Here's the drawing with two shaded views (mm, measured from the low corner). I have some questions. Coordinates: 2 decimals unless noted, no trailing zeros. Loops run counter-clockwise (first coordinate to the right, second up) from the corner with the lowest first, then second, coordinate; pieces in that order, holes last.
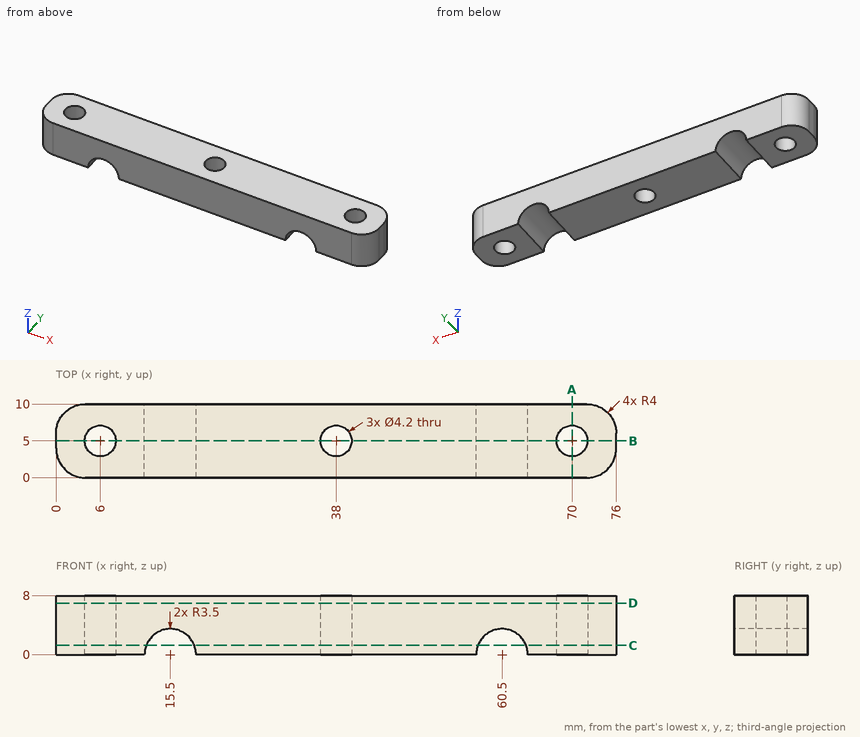
Q1. Suppose I cut it at B-B on y = 5. Write out the boundary of the cut face in (x, z).
Q2. Please list where these lines run through material, in increasing order: probe 1 along Y at (x, z) = (38, 4.75); probe 2 along X at (y, z) = (3.5, 7); probe 3 along X at (y, z) = (1.5, 0.5).
Q3. Suppose I cut it at D-D on z = 7. Write out the boundary of the cut face in (x, y), and give its area (3 significant figures).
Q4. Suppose I cut it at C-C on z = 1.25. Write out the boundary of the cut face in (x, y), and give its area (3 significant figures).
Q5. Suppose I cut it at A-A on x = 70. Write out the boundary of the cut face in (y, z), and give its area (3 significant figures).
Check values:
1. outline: (0, 0) - (3.9, 0) - (3.9, 8) - (0, 8) - close; (8.1, 0) - (12, 0) arc R3.5 cw to (19, 0) - (35.9, 0) - (35.9, 8) - (8.1, 8) - close; (40.1, 0) - (57, 0) arc R3.5 cw to (64, 0) - (67.9, 0) - (67.9, 8) - (40.1, 8) - close; (72.1, 0) - (76, 0) - (76, 8) - (72.1, 8) - close
2. probe 1: y = 0 to 2.9, 7.1 to 10
2. probe 2: x = 0.03 to 4.53, 7.47 to 36.53, 39.47 to 68.53, 71.47 to 75.97
2. probe 3: x = 0.88 to 12.04, 18.96 to 57.04, 63.96 to 75.12
3. outline: (0, 4) arc R4 ccw to (4, 0) - (72, 0) arc R4 ccw to (76, 4) - (76, 6) arc R4 ccw to (72, 10) - (4, 10) arc R4 ccw to (0, 6) - close; hole circle Ø4.2 at (6, 5); hole circle Ø4.2 at (38, 5); hole circle Ø4.2 at (70, 5)
3. area: 705 mm2
4. outline: (0, 4) arc R4 ccw to (4, 0) - (12.23, 0) - (12.23, 10) - (4, 10) arc R4 ccw to (0, 6) - close; (18.77, 0) - (57.23, 0) - (57.23, 10) - (18.77, 10) - close; (63.77, 0) - (72, 0) arc R4 ccw to (76, 4) - (76, 6) arc R4 ccw to (72, 10) - (63.77, 10) - close; hole circle Ø4.2 at (6, 5); hole circle Ø4.2 at (38, 5); hole circle Ø4.2 at (70, 5)
4. area: 574 mm2
5. outline: (0, 0) - (2.9, 0) - (2.9, 8) - (0, 8) - close; (7.1, 0) - (10, 0) - (10, 8) - (7.1, 8) - close
5. area: 46.4 mm2
